Can you work these out from the drawing? Everything is in mm from the part's minimum corner. A direction names the side the tool comes from. Round coordinates to 2 decimals unless told otherwise and drop trailing zeros. Loops run counter-clockwise (first coordinate to the right, second up) from the corner with the lowest first, then second, coordinate; pieces in that order, holes last. Notation, with made-up numbers: (-21, 21.25) -> (-13, 21.25) arc R18 cw to (-13, 43.25) -> close; hole circle Ø1 at (73.25, -18). An arc over 180 degrees is marked (long way). One line per item, written item: value.
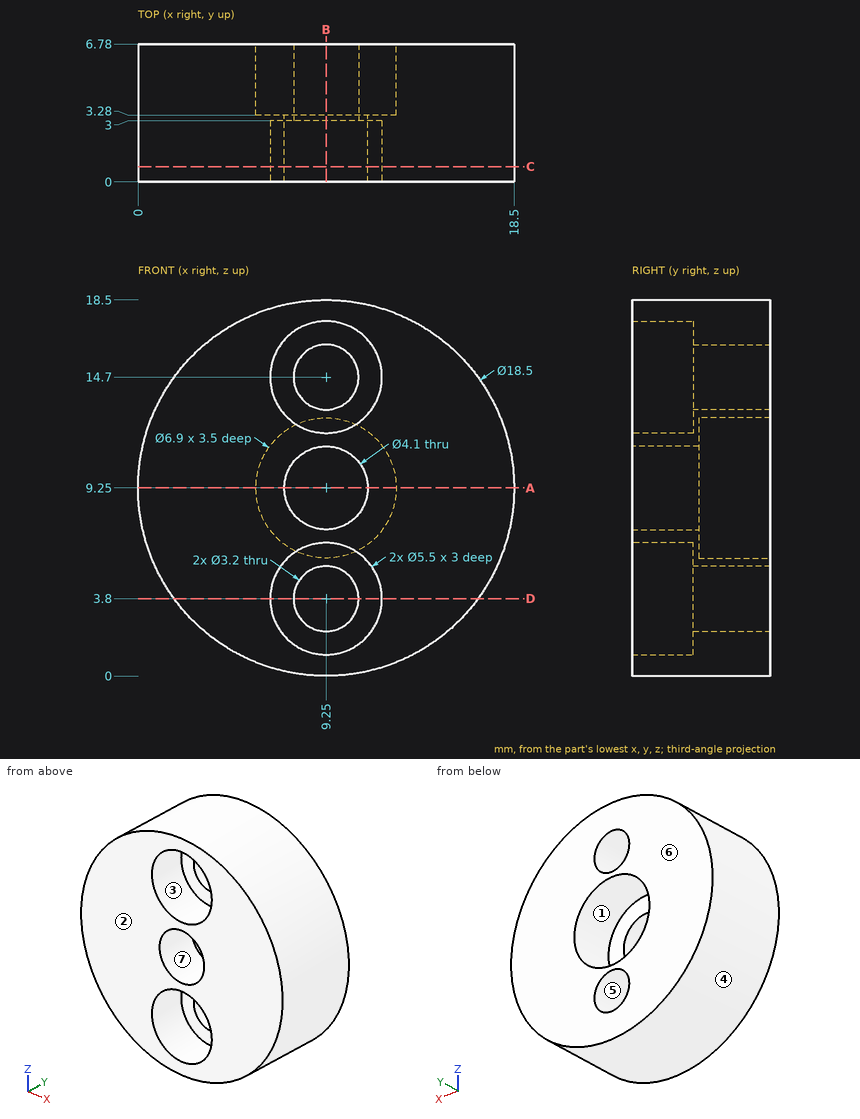
Item 1: If we mould it in two halves opening along Z, with no side actions, what happens to the marked faces 4, 5, 6 and 7? For each: released by +Z, released by -Z, zero draft, split by the parting line, or undercut.
Output:
face 4: split by the parting line
face 5: undercut
face 6: zero draft
face 7: undercut
Item 2: If we section it at C-C on y = 0.75: List the corners of the cut face in (x, z) for me.
Output:
outline: circle Ø18.5 at (9.25, 9.25); hole circle Ø5.5 at (9.25, 3.8); hole circle Ø5.5 at (9.25, 14.7); hole circle Ø4.1 at (9.25, 9.25)
Item 3: Will these pins go through, and if not, where does the flat tip stop? pin 1 Ø5.5 at (x, z) = (9.25, 9.25) entering from +Y; pin 2 Ø1.5 at (y, z) = (4.5, 13) entering from -X; pin 3 Ø1.5 at (x, z) = (9, 15) entering from +Y; pin 4 Ø3.5 at (x, z) = (9.25, 3.8) entering from -Y.
Output:
pin 1: stops at y = 3.28
pin 2: stops at x = 0.5
pin 3: passes through
pin 4: stops at y = 3
Item 4: I need wall thicknesses on line 1 (X direction, y = 5.65, z = 9.25); line 2 (X direction, y = 0.75, z = 3.25); line 3 (Z direction, x = 7, y = 1.75). Which ranges of each line are inside material? Lowest first, please. Write a range as from..to.
Output:
line 1: x = 0..5.8, 12.7..18.5
line 2: x = 2.21..6.56, 11.94..16.29
line 3: z = 0.28..2.22, 5.38..13.12, 16.28..18.22
Item 5: If we section it at A-A on z = 9.25: List the corners of the cut face in (x, y) for me, plus the area to 3 significant figures.
Output:
outline: (0, 0) -> (7.2, 0) -> (7.2, 3.28) -> (5.8, 3.28) -> (5.8, 6.78) -> (0, 6.78) -> close; (11.3, 0) -> (18.5, 0) -> (18.5, 6.78) -> (12.7, 6.78) -> (12.7, 3.28) -> (11.3, 3.28) -> close
area: 87.8 mm²
Item 6: If we section it at B-B on x = 9.25: List the corners of the cut face in (y, z) for me.
Output:
outline: (0, 0) -> (6.78, 0) -> (6.78, 2.2) -> (3, 2.2) -> (3, 1.05) -> (0, 1.05) -> close; (0, 6.55) -> (3, 6.55) -> (3, 5.4) -> (6.78, 5.4) -> (6.78, 5.8) -> (3.28, 5.8) -> (3.28, 7.2) -> (0, 7.2) -> close; (0, 11.3) -> (3.28, 11.3) -> (3.28, 12.7) -> (6.78, 12.7) -> (6.78, 13.1) -> (3, 13.1) -> (3, 11.95) -> (0, 11.95) -> close; (0, 17.45) -> (3, 17.45) -> (3, 16.3) -> (6.78, 16.3) -> (6.78, 18.5) -> (0, 18.5) -> close
Item 7: If we section it at D-D on z = 3.8: List the corners of the cut face in (x, y) for me.
Output:
outline: (1.78, 0) -> (6.5, 0) -> (6.5, 3) -> (7.65, 3) -> (7.65, 6.78) -> (1.78, 6.78) -> close; (10.85, 3) -> (12, 3) -> (12, 0) -> (16.72, 0) -> (16.72, 6.78) -> (10.85, 6.78) -> close
Item 8: For the marked faces 1, 2 and 3, which set-ups out of +Z, -Z, +X, -X, +Y, -Y let a thin tool reach every point of the face, with its end or its side?
Output:
face 1: +Y
face 2: +Z, -Z, +X, -X, -Y
face 3: -Y
